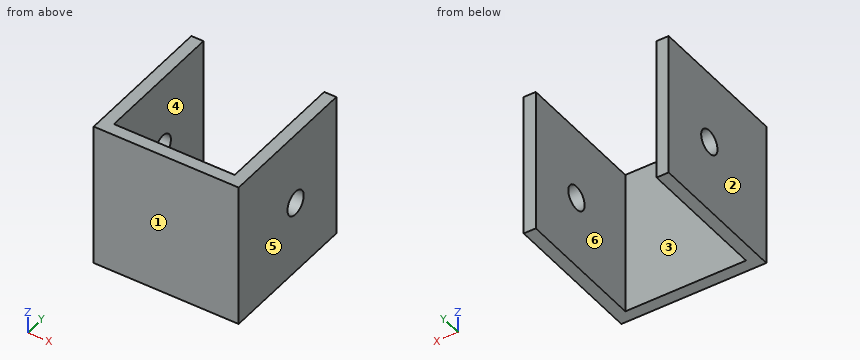
Autodesk Inventor part; units mm, degrees
ref_plane "YZ Plane" through (0, 0, 0) normal (1, 0, 0) x (0, 1, 0)
ref_plane "XZ Plane" through (0, 0, 0) normal (0, 1, 0) x (-1, 0, 0)
ref_plane "XY Plane" through (0, 0, 0) normal (0, 0, 1) x (1, 0, 0)
sketch "Sketch1" plane through (0, 0, 0) normal (0, 0, 1) x (1, 0, 0)
  line L0 (0, 0) -> (0, 38.1)
  line L1 (0, 38.1) -> (3.175, 38.1)
  line L2 (3.175, 38.1) -> (3.175, 3.175)
  line L3 (3.175, 3.175) -> (34.925, 3.175)
  line L4 (34.925, 3.175) -> (34.925, 38.1)
  line L5 (34.925, 38.1) -> (38.1, 38.1)
  line L6 (38.1, 38.1) -> (38.1, 0)
  line L7 (38.1, 0) -> (0, 0)
  dimension "d0" = 38.1
  dimension "d2" = 3.175
  dimension "d3" = 3.175
  dimension "d4" = 38.1
  dimension "d5" = 3.175
extrude "Extrusion1" add sketch "Sketch1" along normal blind 38.1
sketch "Sketch2" plane through (38.1, 0, 0) normal (1, 0, 0) x (0, 0, -1)
  line L0 (0, 38.1) -> (0, 0)
  line L1 (0, 38.1) -> (-38.1, 38.1)
  line L2 (-38.1, 0) -> (-38.1, 38.1)
  line L3 (0, 0) -> (-38.1, 0)
  line L4 (0, 3.175) -> (-38.1, 3.175)
  point P0 (0, 0)
  point P1 (-19.05, 22.225)
  dimension "d8" = 19.05
  dimension "d9" = 19.05
  dimension "d19" = 19.05
hole "Hole1" at (38.1, 22.225, 19.05) direction (-1, 0, 0) diameter 6.35 end through all
equation "\"d3\" = d2"
equation "\"d5\" = d2"
properties part number "CLB_062_ScissorLiftUBracket"
Verification items for the finished model (mm, model axes). Face numbers are marked on the shaded views. A direction names the side the tool comes from. Give positions to 0.01 mm unless a question says otherwise; leave off trailing zeros. Order: outer loops, then holes, each group sorted by start corner. A loop starts at its lowest first (then second) coordinate and runs counter-clockwise, first axis right, second up. Notation, with made-up numbers: M 43.25,58 L 95.25,58 A26 cw 95.25,85 Z; hole C 37,19.25 d6. An arc over 180 degrees is marked long. Answer as a JSON object with one key per item and string values. Group by question number.
1) Scan lines: line 1 along X through (y, z) = (35, 19) (3 decimals); line 2 along Y through (x, z) = (36, 19); line 3 along Y through (x, z) = (21, 20.5) (3 decimals). Record each from-to range of solid material in increasing order. Write a range as [from, to].
2) Cross-section at C-C (y = 23). Enter the section's corners in (x, z) (3 decimals), then the cut area to 3 significant figures.
3) Cross-section at D-D (z = 13.5). Enter the section's corners in (x, y) (3 decimals).
4) Cross-section at A-A (y = 35.5). Enter the section's corners in (x, z) (3 decimals), then the cut area to 3 significant figures.
5) Access from +Z, -Z, +X, -X, +Y, -Y to the whole of each face (thin tool, end or side, straight path). Record for the marked faces 5 and 6.
6) Cross-section at B-B (z = 19.05). Enter the section's corners in (x, y) (3 decimals), then the cut area to 3 significant figures.
7) Depth check by flat-ended pin: pin 1 Ø4 at (y, z) = (29, 7) entering from -X; pin 2 Ø5 at (x, z) = (10, 20) entering from +Y (3 decimals). Enter the tip coordinate at first touch or a pass-through.
8) Mould release check, pull along X, two halves, no side actions. Record for the marked faces 1, 2, 3 and 4: released by +X, released by -X, zero draft, split by the parting line, or undercut.
Result sheet:
{
 "1": {"line 1": "x = [0, 3.175], [34.925, 38.1]", "line 2": "y = [0, 19.05], [25.4, 38.1]", "line 3": "y = [0, 3.175]"},
 "2": {"outline": "M 0,0 L 3.175,0 L 3.175,15.971 L 0,15.971 Z; M 0,22.129 L 3.175,22.129 L 3.175,38.1 L 0,38.1 Z; M 34.925,0 L 38.1,0 L 38.1,15.971 L 34.925,15.971 Z; M 34.925,22.129 L 38.1,22.129 L 38.1,38.1 L 34.925,38.1 Z", "area": "203 mm2"},
 "3": {"outline": "M 0,0 L 38.1,0 L 38.1,38.1 L 34.925,38.1 L 34.925,3.175 L 3.175,3.175 L 3.175,38.1 L 0,38.1 Z"},
 "4": {"outline": "M 0,0 L 3.175,0 L 3.175,38.1 L 0,38.1 Z; M 34.925,0 L 38.1,0 L 38.1,38.1 L 34.925,38.1 Z", "area": "242 mm2"},
 "5": {"face 5": "+Z, -Z, +X, +Y, -Y", "face 6": "+Z, -Z, +Y"},
 "6": {"outline": "M 0,0 L 38.1,0 L 38.1,19.05 L 34.925,19.05 L 34.925,3.175 L 3.175,3.175 L 3.175,19.05 L 0,19.05 Z; M 0,25.4 L 3.175,25.4 L 3.175,38.1 L 0,38.1 Z; M 34.925,25.4 L 38.1,25.4 L 38.1,38.1 L 34.925,38.1 Z", "area": "302 mm2"},
 "7": {"pin 1": "stops at x = 0", "pin 2": "stops at y = 3.175"},
 "8": {"face 1": "zero draft", "face 2": "released by -X", "face 3": "undercut", "face 4": "undercut"}
}
